Can you work these out from the drawing? Everything is in mm from the part's minimum corner. Coordinates: 2 decimals unless noted, no trailing zeros. Order: outer loops, then holes, each group sorted by start corner. A loop starts at its lowest first (then second) coordinate and runs counter-clockwise, first axis right, second up. Notation, with made-up numbers: (81.5, 33) - (125.5, 33) arc R14 ccw to (125.5, 47) - close; hole circle Ø3 at (80.5, 66.25). An arc over 180 degrees is marked (long way). Use a Markdown table: item, result. Add a question column.
(1) I want a section at A-A (x = 0.55). List the corners of the cut face in (y, z) for me.
(2) For pin 1 Ø2 at (y, z) = (5.5, 4) entering from +X; pin 2 Ø1.5 at (y, z) = (9, 5.5) entering from +X; pin 3 Ø1.6 at (x, z) = (3.5, 2) entering from +Y; pin 4 Ø1.5 at (y, z) = (12.5, 5) entering from -X, each with a flat end and sliding along its axis, tell me the tip position at first contact or that it passes through.
(3) If I drill on L1, parallel to Z at x = 2.75, y = 18.5 (1 decimal); L2, parallel to Y at x = 4.85, z = 1.25; L3, parallel to X at y = 13.75, z = 3.25, over which ranges is the centre line in solid material (lowest first)? Write a range as [from, to].
(4) We'd pull the mould along Z, two halves only. Please class the marked faces 1, 2 and 3: pulls with the +Z half, pulls with the -Z half, needs draft (parallel to the pull), parting line crosses it, or undercut.
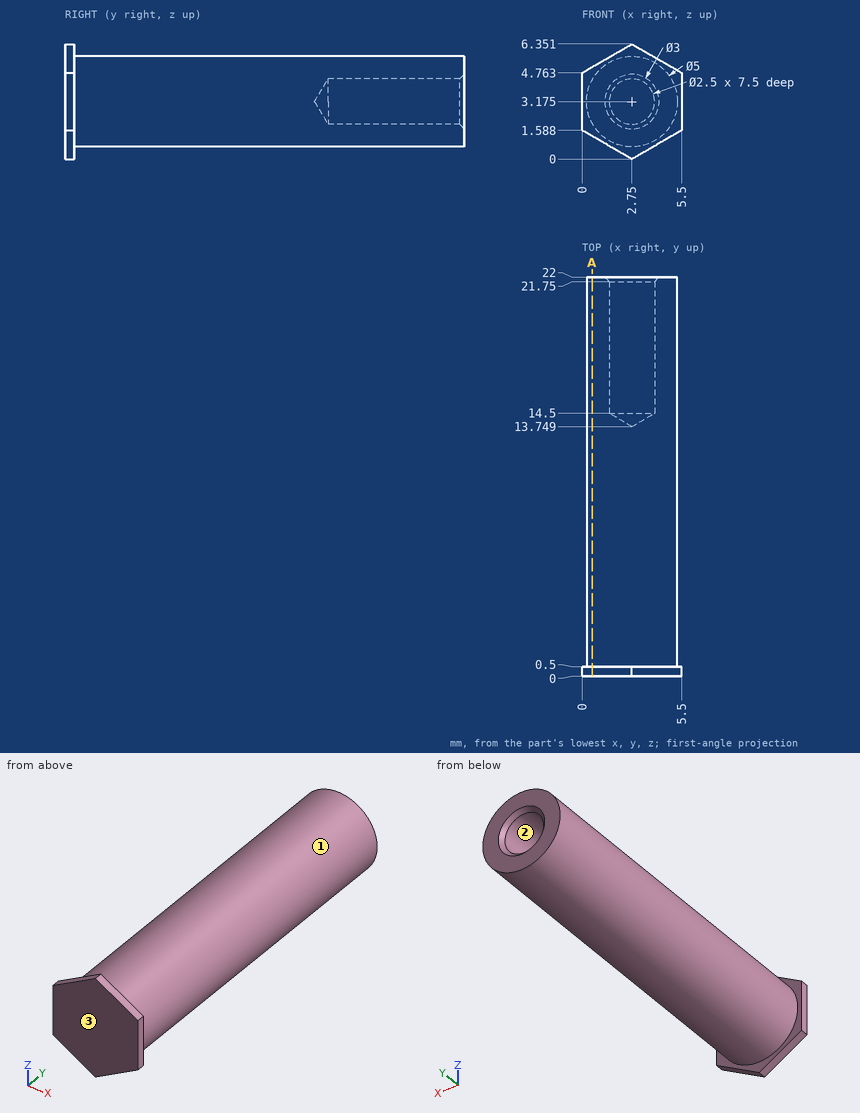
Answers follow:
| question | item | result |
|---|---|---|
| 1 | outline | (0, 1.27) - (0.5, 1.27) - (0.5, 1.99) - (22, 1.99) - (22, 4.36) - (0.5, 4.36) - (0.5, 5.08) - (0, 5.08) - close |
| 2 | pin 1 | stops at x = 5.25 |
| 2 | pin 2 | stops at x = 4.69 |
| 2 | pin 3 | stops at y = 22 |
| 2 | pin 4 | stops at x = 0.49 |
| 3 | L1 | z = [0.7, 1.9], [4.4, 5.7] |
| 3 | L2 | y = [0, 0.5] |
| 3 | L3 | x = [0.25, 5.25] |
| 4 | face 1 | parting line crosses it |
| 4 | face 2 | undercut |
| 4 | face 3 | needs draft |
